Read the model definition and answer for the solid it produces. Units are mm, in the model's axes. Face numbers are marked on the shaded views. A direction names the side the tool comes from. Give positions to 0.01 mm unless a question says otherwise; leave off trailing zeros. Loops run counter-clockwise (first coordinate to the right, second up) from the corner with the lowest first, then second, coordinate; pieces in that order, holes last. Notation, with made-up numbers: (6, 74) - (32, 74) arc R17 cw to (32, 78) - close; hole circle Ø7 at (12, -4). An arc over 180 degrees is marked (long way). Write item = value, one per line.
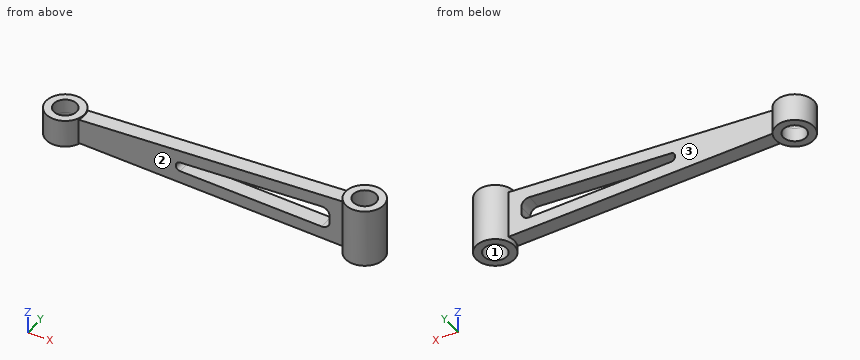
```python
from build123d import *

# Parameters (mm, degrees)
SKETCH1_R           = 12.5
BOSS_EXTRUDE1_DEPTH = 9
SKETCH2_R           = 12.5
BOSS_EXTRUDE2_DEPTH = 19
BOSS_EXTRUDE3_DEPTH = 5
CUT_EXTRUDE1_DEPTH  = 26.5
SKETCH5_R           = 7.5
CUT_EXTRUDE2_DEPTH  = 26.5


with BuildPart() as part:
    # Sketch1 → Boss-Extrude1 (new, symmetric)
    with BuildSketch(Plane.XY):
        with Locations((-97.28, 0)):
            Circle(SKETCH1_R)
    extrude(amount=BOSS_EXTRUDE1_DEPTH, both=True)



with BuildPart() as body_2:
    # Sketch2 → Boss-Extrude2 (new, symmetric)
    with BuildSketch(Plane.XY):
        with Locations((97.28, 0)):
            Circle(SKETCH2_R)
    extrude(amount=BOSS_EXTRUDE2_DEPTH, both=True)


with BuildPart() as part_1:
    add(part.part)

    add(body_2.part)  # Boss-Extrude3 merges body 2
    # Sketch3 → Boss-Extrude3 (add, symmetric)
    with BuildSketch(Plane(origin=(0, 0, 0), x_dir=(1, 0, 0), z_dir=(0, 1, 0))):
        Polygon((-97.28, 7.645187817), (97.28, 16.139860869), (97.28, -16.139860869), (-97.28, -7.645187817), align=None)
    extrude(amount=BOSS_EXTRUDE3_DEPTH, both=True)

    # Sketch4 → Cut-Extrude1 (cut, symmetric)
    with BuildSketch(Plane(origin=(0, 5, 0), x_dir=(1, 0, 0), z_dir=(0, 1, 0))):
        with BuildLine():
            Line((72.223918829, 7.038267258), (-19.688842396, 3.025269438))
            ThreePointArc((-19.688842396, 3.025269438), (-21.72507612, 2.102663941), (-22.557984234, 0.028124773))
            Line((-22.557984234, 0.028124773), (-22.557984234, -0.028124773))
            ThreePointArc((-22.557984234, -0.028124773), (-21.72507612, -2.102663941), (-19.688842396, -3.025269438))
            Line((-19.688842396, -3.025269438), (72.223918829, -7.038267258))
            ThreePointArc((72.223918829, -7.038267258), (75.899581045, -5.654845961), (77.442015766, -2.04302615))
            Line((77.442015766, -2.04302615), (77.442015766, 2.04302615))
            ThreePointArc((77.442015766, 2.04302615), (75.899581045, 5.654845961), (72.223918829, 7.038267258))
        make_face()
    extrude(amount=CUT_EXTRUDE1_DEPTH, both=True, mode=Mode.SUBTRACT)

    # Sketch5 → Cut-Extrude2 (cut, symmetric)
    with BuildSketch(Plane.XY):
        with Locations((-97.28, 0)):
            Circle(SKETCH5_R)
        with Locations((97.28, 0)):
            Circle(SKETCH5_R)
    extrude(amount=CUT_EXTRUDE2_DEPTH, both=True, mode=Mode.SUBTRACT)


solid = part_1.part
```
1) A cutting plane is placed at B-B on y = 10. Determine the outline of the cut face in (x, z), then the cut area to 3 significant figures.
Output:
outline = (-104.78, -9) - (-89.78, -9) - (-89.78, 9) - (-104.78, 9) - close; (89.78, -19) - (104.78, -19) - (104.78, 19) - (89.78, 19) - close
area = 840 mm²
2) A tool of negligible diameter and unlimited length cuts with its end or side. For the marked faces 1, 2 and 3, from which of +Z, -Z, +X, -X, +Y, -Y can it reach the whole face along a straight path? Write none if from no direction.
Output:
face_1 = +Z, -Z
face_2 = +Z, -Z, -Y
face_3 = +Z, -Z, +Y
3) A cutting plane is placed at D-D on x = -71.5. Determine the outline of the cut face in (y, z).
Output:
outline = (-5, -8.77) - (5, -8.77) - (5, 8.77) - (-5, 8.77) - close
4) A cutting plane is placed at C-C on z = 13.5. Determine the outline of the cut face in (x, y).
Output:
outline = (36.82, -5) - (85.82, -5) arc R12.5 ccw (long way) to (85.82, 5) - (36.82, 5) - close; hole circle Ø15 at (97.28, 0)
5) Each of these flat-tipped pins is pushed along its axis until it touches: P1, Ø8, axis at x = -71.5, z = 4, coming from the -Y side; P2, Ø12, axis at x = 28.5, z = -1.5, coming from the +Y side; P3, Ø7.5, axis at x = -95, y = 1, coming from the -Z side; P4, Ø5, axis at x = 4, y = 6, coming from the -Z side. Where does it stop, or does it pass through?
Output:
P1 = -5
P2 = 5
P3 = through
P4 = -12.17
6) A cutting plane is placed at A-A on x = -97.28. Determine the outline of the cut face in (y, z), then the cut area to 3 significant figures.
Output:
outline = (-12.5, -9) - (-7.5, -9) - (-7.5, 9) - (-12.5, 9) - close; (7.5, -9) - (12.5, -9) - (12.5, 9) - (7.5, 9) - close
area = 180 mm²
7) Find the intervals of material crossed by probe 1 along Y at (x, z) = (97, -2); probe 2 along Z at (x, y) = (-99.5, 9.75); probe 3 along X at (y, z) = (2.25, -0.5), in increasing order.
Output:
probe_1 = -12.5 to -7.49, 7.49 to 12.5
probe_2 = -9 to 9
probe_3 = -109.58 to -104.43, -90.13 to -22.52, 77.44 to 90.13, 104.43 to 109.58
